Source: CAD feature listing. Evaluate the final solid. Frame: model axes, mm. A direction names the side the tool comes from. Give positions to 0.01 mm unless a question says otherwise; leave off trailing zeros. Order: outer loops, then holes, each group sorted by start corner. A loop starts at its lowest first (then second) coordinate and runs counter-clockwise, first axis right, second up.
1) Section C-C, the plane y = 29.5. Return loops of the section in (x, z).
2) Draft query along Y for faces 1 (the face through (0, 0, 2)), 2 (the face through (-10, 50, 2)), 3 (the face through (-6, 28, 0)). Return one class per face: released by +Y, released by -Y, zero draft, split by the parting line, or undercut.
3) Section B-B, the plane z = 2.2. Give the number of separate pieces and of enclosed holes in the cut face, plus the area to 3 significant figures.
4) First-contact query: P1, Ø2.5, axis at x = 10, z = 1.5, coming from the +Y side; P2, Ø1.5, axis at x = -10, z = 3, coming from the +Y side; P3, Ø1.5, axis at y = 47.5, z = 3, coming from the -X side. Flat tips, straight axial feed; report the tip coordinate or a pass-through.
5) Material intervals for line 1 (Y direction, x = 0, z = 2.55); line 2 (Y direction, x = -0.75, z = 3.5); line 3 (Y direction, x = 8, z = 3.15), sorted ascending.
6) Section D-D, the plane y = 7.5. Return loops of the section in (x, z).
7) Section A-A, the plane x = 0. Return loops of the section in (y, z), plus the area to 4 significant figures.
8) Access query for faces 4 (the face through (0, 55, 2)), 5 (the face through (10, 50, 2)), 6 (the face through (-7.5, 48, 2)). Directions: +Z, -Z, +X, -X, +Y, -Y. A direction counts if a zero-diameter tool reaches every point of the face in a straight line with its end or side. Return the directions, or none.
```python
from build123d import *

# Parameters (mm, degrees)
ESQUISSE1_R        = 1.5
ESQUISSE1_R_2      = 4.25
BOSS_EXTRU_1_DEPTH = 5
CONG_1_R           = 5


with BuildPart() as part:
    # Esquisse1 → Boss.-Extru.1 (new body)
    with BuildSketch(Plane.XY):
        Polygon((-12.5, 0), (12.5, 0), (12.5, 5), (7.5, 5), (7.5, 10), (12.5, 10), (12.5, 45), (7.5, 45), (7.5, 50), (12.5, 50), (12.5, 55), (-12.5, 55), (-12.5, 50), (-7.5, 50), (-7.5, 45), (-12.5, 45), (-12.5, 10), (-7.5, 10), (-7.5, 5), (-12.5, 5), align=None)
        with Locations((0, 47.5)):
            Circle(ESQUISSE1_R, mode=Mode.SUBTRACT)
        with Locations((0, 7.5)):
            Circle(ESQUISSE1_R, mode=Mode.SUBTRACT)
        with Locations((0, 27.5)):
            Circle(ESQUISSE1_R_2, mode=Mode.SUBTRACT)
    extrude(amount=BOSS_EXTRU_1_DEPTH)

    # Congé1
    cong_1_edges = [part.edges().sort_by_distance(p)[0] for p in [
        (12.5, 55, 2.5),
        (12.5, 0, 2.5),
        (-12.5, 0, 2.5),
        (-12.5, 55, 2.5),
    ]]
    fillet(cong_1_edges, radius=CONG_1_R - 0.0001)  # a hair under: the kernel refuses the full size


solid = part.part
```
From the geometry:
1. outline: (-12.5, 0) - (-3.75, 0) - (-3.75, 5) - (-12.5, 5) - close; (3.75, 0) - (12.5, 0) - (12.5, 5) - (3.75, 5) - close
2. face 1: released by -Y
2. face 2: undercut
2. face 3: zero draft
3. separate pieces: 1
3. enclosed holes: 3
3. area: 1,180 mm2
4. P1: stops at y = 54.84
4. P2: stops at y = 54.68
4. P3: stops at x = -7.5
5. line 1: y = 0 to 6, 9 to 23.25, 31.75 to 46, 49 to 55
5. line 2: y = 0 to 6.2, 8.8 to 23.32, 31.68 to 46.2, 48.8 to 55
5. line 3: y = 0.03 to 5, 10 to 45, 50 to 54.97
6. outline: (-7.5, 0) - (-1.5, 0) - (-1.5, 5) - (-7.5, 5) - close; (1.5, 0) - (7.5, 0) - (7.5, 5) - (1.5, 5) - close
7. outline: (0, 0) - (6, 0) - (6, 5) - (0, 5) - close; (9, 0) - (23.25, 0) - (23.25, 5) - (9, 5) - close; (31.75, 0) - (46, 0) - (46, 5) - (31.75, 5) - close; (49, 0) - (55, 0) - (55, 5) - (49, 5) - close
7. area: 202.5 mm2
8. face 4: +Z, -Z, +X, -X, +Y
8. face 5: +Z, -Z, +X
8. face 6: +Z, -Z, -X
